Input: part model. Units: mm. Frame: model coordinates. Face numbers are marked on the shaded views. Give positions to 0.01 mm unless a question says otherwise; leave off trailing zeros. Loops run counter-clockwise (first coordinate to the right, second up) from the corner with the lowest first, then second, coordinate; pieces in that order, holes last. Notation, with made-up numbers: M -4,40 L 32,40 A15 cw 32,48 Z; hole C 38.25,-2 d8. An arc over 180 degrees is marked long. Use CSV: the item, a comma, the result in double quotes. Start each with the question number.
Q1. Material intervals for line 1 along Y through (x, z) = (0, 31) (3 decimals); line 2 along Z through (x, y) = (7, -75.5); line 3 along Y through (x, z) = (-18, 67.5), sorted ascending.
Q2. Section C-C, the plane z = 6. Output: boundary loops of the cut face in (x, y) (3 decimals).
Q3. Pin query (flat end, axial travel): pin 1 (1.5 mm diameter, centred on x = -40.5, z = 20, fed in from +Y); pin 2 (5 mm diameter, centred on x = 58.5, y = -14.5, fed in from +Z); pin 3 (10 mm diameter, centred on x = 23.5, z = 37, fed in from -Y) (3 decimals). Return the tip coordinate at first contact, or that it passes through.
Q4. Section A-A, the plane y = 0. Output: boundary loops of the cut face in (x, z) (3 decimals), plus the area to 3 significant figures.
Q5. Section D-D, the plane z = 57. Output: boundary loops of the cut face in (x, y) (3 decimals).
Q6. Pull-direction query (Y, two-part tool) for the marked faces 1, 2 and 3; classes: released by +Y, released by -Y, zero draft, split by the parting line, or undercut.
from build123d import *

# Parameters (mm, degrees)
F0_R     = 79.375
F1_DEPTH = 12.7
F0_R_2   = 85.725
F2_DEPTH = 76.2
F3_R     = 1.27
F4_R     = 0.254


with BuildPart() as f1:
    # F0 (on Top) → F1 (new body)
    with BuildSketch(Plane.XY):
        Circle(F0_R)
    extrude(amount=F1_DEPTH)

    # F0 (on Top) → F2 (join)
    with BuildSketch(Plane.XY):
        Circle(F0_R_2)
        Circle(F0_R, mode=Mode.SUBTRACT)
    extrude(amount=F2_DEPTH)

    # F3
    f3_edges = [f1.edges().sort_by_distance(p)[0] for p in [
        (-85.725, 0, 0),
        (-79.375, 0, 12.7),
    ]]
    fillet(f3_edges, radius=F3_R)

    # F4
    f4_edges = [f1.edges().sort_by_distance(p)[0] for p in [
        (-79.375, 0, 76.2),
        (-85.725, 0, 76.2),
    ]]
    fillet(f4_edges, radius=F4_R)


solid = f1.part
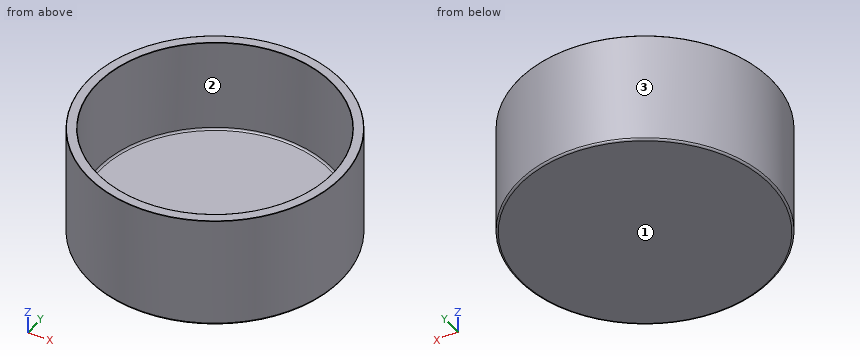
A:
1,line 1,"-85.725 to -79.375, 79.375 to 85.725"
1,line 2,"0 to 12.7"
1,line 3,"-83.81 to -77.31, 77.31 to 83.81"
2,outline,"C 0,0 d171.45"
3,pin 1,"y = 75.95"
3,pin 2,"z = 12.7"
3,pin 3,"y = -83.705"
4,outline,"M -85.725,1.27 A1.27 ccw -84.455,0 L 84.455,0 A1.27 ccw 85.725,1.27 L 85.725,75.946 A0.254 ccw 85.471,76.2 L 79.629,76.2 A0.254 ccw 79.375,75.946 L 79.375,13.97 A1.27 cw 78.105,12.7 L -78.105,12.7 A1.27 cw -79.375,13.97 L -79.375,75.946 A0.254 ccw -79.629,76.2 L -85.471,76.2 A0.254 ccw -85.725,75.946 Z"
4,area,"2,980 mm^2"
5,outline,"C 0,0 d171.45; hole C 0,0 d158.75"
6,face 1,"zero draft"
6,face 2,"undercut"
6,face 3,"split by the parting line"
